from build123d import *

# Parameters (mm, degrees)
SKETCH1_W           = 100
SKETCH1_H           = 100
BOSS_EXTRUDE1_DEPTH = 3
SKETCH4_R           = 1.7
CUT_EXTRUDE3_DEPTH  = 3
SKETCH2_W           = 10
SKETCH2_H           = 38
CUT_EXTRUDE4_DEPTH  = 3
SKETCH5_R           = 1.8
SKETCH5_R_2         = 1.7
SKETCH5_W           = 12
SKETCH5_H           = 4
SKETCH5_W_2         = 4
SKETCH5_H_2         = 12
CUT_EXTRUDE5_DEPTH  = 3
FILLET1_R           = 10
FILLET2_R           = 3
FILLET3_R           = 10
FILLET4_R           = 3
FILLET5_R           = 3
FILLET6_R           = 1


with BuildPart() as part:
    # Sketch1 → Boss-Extrude1 (new body)
    with BuildSketch(Plane(origin=(0, 0, 0), x_dir=(1, 0, 0), z_dir=(0, 1, 0))):
        Rectangle(SKETCH1_W, SKETCH1_H)
    extrude(amount=BOSS_EXTRUDE1_DEPTH)

    # Sketch4 → Cut-Extrude3 (cut)
    with BuildSketch(Plane(origin=(0, 3, 0), x_dir=(1, 0, 0), z_dir=(0, 1, 0))):
        with Locations(Location((-41, 20, 0), (0, 0, 270))):
            Circle(SKETCH4_R)
        with Locations(Location((-41, -41, 0), (0, 0, 270))):
            Circle(SKETCH4_R)
        with Locations(Location((41, -41, 0), (0, 0, 270))):
            Circle(SKETCH4_R)
        with Locations(Location((41, 20, 0), (0, 0, 270))):
            Circle(SKETCH4_R)
    extrude(amount=-CUT_EXTRUDE3_DEPTH, mode=Mode.SUBTRACT)

    # Sketch2 → Cut-Extrude4 (cut)
    with BuildSketch(Plane(origin=(0, 3, 0), x_dir=(1, 0, 0), z_dir=(0, 1, 0))):
        with Locations((-45, -13)):
            Rectangle(SKETCH2_W, SKETCH2_H)
    cut_extrude4 = extrude(amount=-CUT_EXTRUDE4_DEPTH, mode=Mode.SUBTRACT)

    # Mirror2: Cut-Extrude4 across plane
    add(cut_extrude4.mirror(Plane(origin=(0, 0, 0), x_dir=(0, 0, 1), z_dir=(1, 0, 0))), mode=Mode.SUBTRACT)

    # Sketch5 → Cut-Extrude5 (cut)
    with BuildSketch(Plane(origin=(0, 3, 0), x_dir=(1, 0, 0), z_dir=(0, 1, 0))):
        with Locations(Location((-32, -0.5, 0), (0, 0, 270))):
            Circle(SKETCH5_R)
        with Locations(Location((-32, -25.5, 0), (0, 0, 270))):
            Circle(SKETCH5_R)
        with Locations(Location((32, -25.5, 0), (0, 0, 270))):
            Circle(SKETCH5_R)
        with Locations(Location((32, -0.5, 0), (0, 0, 270))):
            Circle(SKETCH5_R)
        with Locations(Location((-21.5, 39, 0), (0, 0, 270))):
            Circle(SKETCH5_R_2)
        with Locations(Location((21.5, 39, 0), (0, 0, 270))):
            Circle(SKETCH5_R_2)
        with Locations((0, -5)):
            Rectangle(SKETCH5_W, SKETCH5_H)
        with Locations((0, 27.5)):
            Rectangle(SKETCH5_W, SKETCH5_H)
        with Locations((-27, 12)):
            Rectangle(SKETCH5_W_2, SKETCH5_H_2)
        with Locations((27, 12)):
            Rectangle(SKETCH5_W_2, SKETCH5_H_2)
    extrude(amount=-CUT_EXTRUDE5_DEPTH, mode=Mode.SUBTRACT)

    # Fillet1
    fillet1_edges = [part.edges().sort_by_distance(p)[0] for p in [
        (-50, 1.5, 50),
        (50, 1.5, 50),
    ]]
    fillet(fillet1_edges, radius=FILLET1_R)

    # Fillet2
    fillet2_edges = [part.edges().sort_by_distance(p)[0] for p in [
        (50, 1.5, -6),
        (50, 1.5, 32),
    ]]
    fillet(fillet2_edges, radius=FILLET2_R)

    # Fillet3
    fillet3_edges = [part.edges().sort_by_distance(p)[0] for p in [
        (-50, 1.5, -50),
        (50, 1.5, -50),
    ]]
    fillet(fillet3_edges, radius=FILLET3_R)

    # Fillet4
    fillet4_edges = [part.edges().sort_by_distance(p)[0] for p in [
        (-50, 1.5, 32),
    ]]
    fillet(fillet4_edges, radius=FILLET4_R)

    # Fillet5
    fillet5_edges = [part.edges().sort_by_distance(p)[0] for p in [
        (-50, 1.5, -6),
    ]]
    fillet(fillet5_edges, radius=FILLET5_R)

    # Fillet6
    fillet6_edges = [part.edges().sort_by_distance(p)[0] for p in [
        (-29, 1.5, -18),
        (-29, 1.5, -6),
        (-25, 1.5, -6),
        (-25, 1.5, -18),
        (25, 1.5, -18),
        (25, 1.5, -6),
        (29, 1.5, -6),
        (29, 1.5, -18),
        (-6, 1.5, 3),
        (-6, 1.5, 7),
        (6, 1.5, 7),
        (6, 1.5, 3),
        (-6, 1.5, -29.5),
        (-6, 1.5, -25.5),
        (6, 1.5, -25.5),
        (6, 1.5, -29.5),
    ]]
    fillet(fillet6_edges, radius=FILLET6_R)


solid = part.part
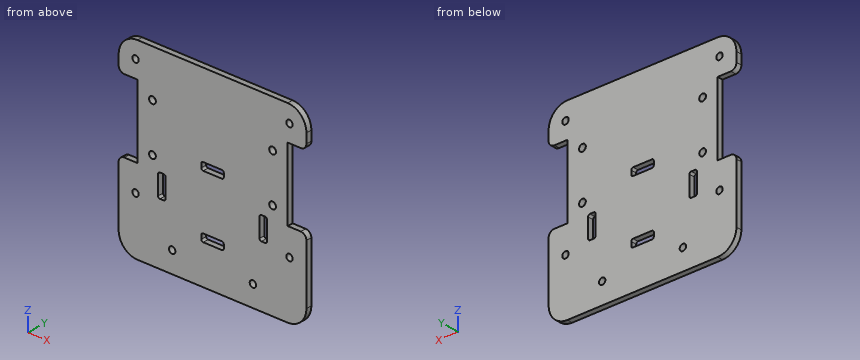
Work out the finished part from the listing and answer in its coordinate system (mm). Round coordinates to 2 decimals unless told otherwise and drop trailing zeros. Write each loop counter-clockwise with the first axis right and the second up, starting at its lowest first coordinate (ties: lowest second). Pieces come first, ordered by that corner, then holes. Notation, with made-up numbers: (60, 74.25) - (66, 74.25) arc R26 cw to (66, 113.25) - close; hole circle Ø9 at (-22, -2). An arc over 180 degrees is marked (long way). Answer in a Markdown table with one row per item. Add a question column.
1. A cutting plane is placed at C-C, the plane y = 2.55. Count the separate pieces of the cut face and the enclosed holes in it, and give its area (3 significant figures).
2. A cutting plane is placed at D-D, the plane z = -38.5. Determine the outline of the cut face in (x, y).
3. A cutting plane is placed at B-B, the plane z = -13. Determine the outline of the cut face in (x, y).
4. Find the intervals of material crossed by line 1 along X through (y, z) = (1.85, -39); line 2 along X through (y, z) = (1.6, -20); line 3 along Z through (x, y) = (1, 2.45), in increasing order. Write a range as from..to.
5. A cutting plane is placed at A-A, the plane x = 21.5. Determine the outline of the cut face in (y, z), and give its area (3 significant figures).
6. Given pin 1 (3 mm diameter, centred on x = -41, z = 41, fed in from -Y); pin 2 (5.5 mm diameter, centred on x = -41, z = -20, fed in from -Y); pin 3 (1.6 mm diameter, centred on y = 1, z = 5.5, fed in from +X); pin 4 (0.9 mm diameter, centred on x = -43.5, y = 1.5, fed in from -Z), each flat-ended and moving along its own axis, determine where each tip first touches the part or whether it passes through.
Worked out:
| question | item | result |
|---|---|---|
| 1 | separate pieces | 1 |
| 1 | enclosed holes | 14 |
| 1 | area | 8,860 mm^2 |
| 2 | outline | (-50, 0) - (-23.12, 0) - (-23.12, 3) - (-50, 3) - close; (-19.88, 0) - (19.88, 0) - (19.88, 3) - (-19.88, 3) - close; (23.12, 0) - (50, 0) - (50, 3) - (23.12, 3) - close |
| 3 | outline | (-50, 0) - (-29, 0) - (-29, 3) - (-50, 3) - close; (-25, 0) - (25, 0) - (25, 3) - (-25, 3) - close; (29, 0) - (50, 0) - (50, 3) - (29, 3) - close |
| 4 | line 1 | -50..-23.2, -19.8..19.8, 23.2..50 |
| 4 | line 2 | -50..-42.7, -39.3..39.3, 42.7..50 |
| 4 | line 3 | -50..-29.5, -25.5..3, 7..50 |
| 5 | outline | (0, -50) - (3, -50) - (3, -40.7) - (0, -40.7) - close; (0, -37.3) - (3, -37.3) - (3, 50) - (0, 50) - close |
| 5 | area | 290 mm^2 |
| 6 | pin 1 | through |
| 6 | pin 2 | y = 0 |
| 6 | pin 3 | x = 40 |
| 6 | pin 4 | z = -49.52 |
